Autodesk Inventor part; units mm, degrees
ref_plane "YZ Plane" through (0, 0, 0) normal (1, 0, 0) x (0, 1, 0)
ref_plane "XZ Plane" through (0, 0, 0) normal (0, 1, 0) x (-1, 0, 0)
ref_plane "XY Plane" through (0, 0, 0) normal (0, 0, 1) x (1, 0, 0)
ref_plane "Płaszczyzna konstrukcyjna1" through (0, 0, 0) normal (0, 0, 1) x (1, 0, 0)
sketch "Szkic1" plane through (0, 0, 0) normal (0, 0, 1) x (1, 0, 0)
  line L0 (-32.2, -16.4467) -> (-32.2, -4.9467)
  line L1 (-32.2, -4.9467) -> (-22.7, -4.9467)
  line L2 (-22.7, -4.9467) -> (-22.7, -16.4467)
  line L3 (-22.7, -16.4467) -> (-32.2, -16.4467)
  line L4 (-31.95, -5.1967) -> (-22.95, -5.1967)
  line L5 (-22.95, -5.1967) -> (-22.95, -16.1967)
  line L6 (-22.95, -16.1967) -> (-31.95, -16.1967)
  line L7 (-31.95, -16.1967) -> (-31.95, -5.1967)
  circle A0 centre (-27.45, -9.3217) radius 3.125
  point P0 (0, 0)
  dimension "d0" = 9
  dimension "d1" = 11
  dimension "d2" = 6.25
extrude "Wyciągnięcie proste1" add sketch "Szkic1" against normal blind 6.5 and the other way blind 0.5 contours L4 L5 L6 L7
chamfer "Faza1" distance 0.25 angle 45 5 edges at (-27.45, -5.1967, 0.5) (-22.95, -10.6967, 0.5) (-31.95, -10.6967, 0.5) (-27.45, -16.1967, 0.5) (-30.575, -9.3217, 0.5)
sketch "Szkic2" plane through (0, 0, -6.5) normal (0, 0, -1) x (-1, 0, 0)
  circle A0 centre (27.45, -9.3217) radius 1
  circle A1 centre (27.45, -9.3217) radius 0.5
  point P0 (0, 0)
  dimension "d11" = 2
  dimension "d12" = 1
extrude "Wyciągnięcie proste2" add sketch "Szkic2" against normal blind 6.5
fillet "Zaokrąglenie1" radius 0.25 1 edges at (-26.45, -9.3217, 0)
fillet "Zaokrąglenie2" radius 0.25 1 edges at (-26.95, -9.3217, 0)
sketch "Szkic3" plane through (0, 0, -6.5) normal (0, 0, -1) x (-1, 0, 0)
  line L0 (31.95, -5.1967) -> (22.95, -5.1967)
  line L1 (22.95, -5.1967) -> (22.95, -16.1967)
  line L2 (22.95, -16.1967) -> (31.95, -16.1967)
  line L3 (31.95, -16.1967) -> (31.95, -5.1967)
  point P0 (0, 0)
extrude "Wyciągnięcie proste3" add sketch "Szkic3" along normal blind 1
properties part number "AUDIO DC12" material "Tworzywo sztuczne, nieprzezroczyste czarne"
Design review of the part built by this model. Coordinates are the model's own, in mm. A direction names the side the tool comes from. Round coordinates to 2 decimals unless told otherwise and drop trailing zeros. Write each loop counter-clockwise with the first axis right and the second up, starting at its lowest first coordinate (ties: lowest second). Pieces come first, ordered by that corner, then holes.
Item 1: For faces 1 (the flat face through (-27, -11, -7.5)), 2 (the cylindrical face through (-30.57, -9.46, -3.17)), list the 3-axis set-ups (+Z, -Z, +X, -X, +Y, -Y) from which the entire face can be reached by the end or side of a thin tool; tool diameter is ignored.
Item 2: Clearance check with a flat-ended pin moving along its axis: pin 1 Ø3 at (x, y) = (-27, -8) entering from +Z. State where the tip first meets the part, or that it passes through.
Item 3: For probe 1 along Y at (x, z) = (-27.45, -3.25); probe 2 along Y at (x, z) = (-28, -4.75); probe 3 along X at (y, z) = (-9.25, -5.5), list the stretches that pass through material, from the lowest coordinate up.
Item 4: We need section A-A on z = -1.75. Write out the cut boundary in (x, y) (3 decimals), and give its area (3 significant figures).
Returned:
1. face 1: -Z, +X, -X, +Y, -Y
1. face 2: +Z
2. pin 1: stops at z = 0
3. probe 1: y = -16.2 to -12.45, -10.32 to -9.82, -8.82 to -8.32, -6.2 to -5.2
3. probe 2: y = -16.2 to -12.4, -10.16 to -8.49, -6.25 to -5.2
3. probe 3: x = -31.95 to -30.57, -28.45 to -27.94, -26.96 to -26.45, -24.33 to -22.95
4. outline: (-31.95, -16.197) - (-22.95, -16.197) - (-22.95, -5.197) - (-31.95, -5.197) - close; circle Ø2 at (-27.45, -9.322); hole circle Ø6.25 at (-27.45, -9.322); hole circle Ø1 at (-27.45, -9.322)
4. area: 70.7 mm2
